CAD build for the part. Positions are in the model's coordinates, mm. Face numbers are marked on the shaded views. A direction names the side the tool comes from. Round coordinates to 2 decimals unless told otherwise and drop trailing zeros. Loops run counter-clockwise (first coordinate to the right, second up) from the corner with the lowest first, then second, coordinate; pieces in that order, holes last. Notation, with made-up numbers: (20.5, -19) - (62.5, -19) arc R33 cw to (62.5, 14) - close; hole circle Ø5 at (83, 54). An arc over 180 degrees is marked (long way). One line per question, with ' | ' between items.
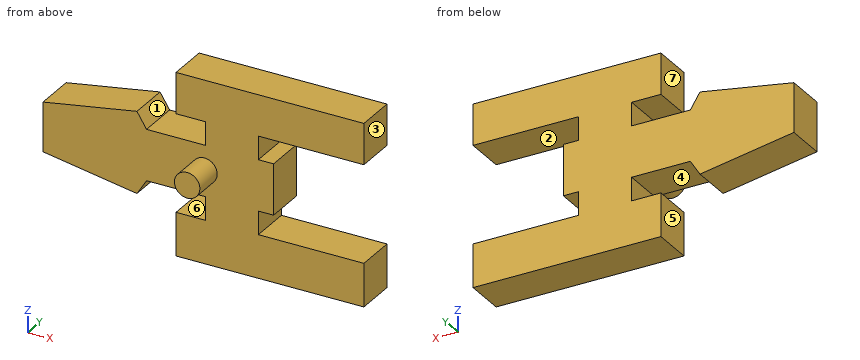
```python
from build123d import *

# Parameters (mm, degrees)
BOSS_EXTRUDE1_DEPTH = 8
SKETCH2_R           = 2.5
BOSS_EXTRUDE2_DEPTH = 6


with BuildPart() as part:
    # Sketch1 → Boss-Extrude1 (new body)
    with BuildSketch(Plane(origin=(0, 0, 0), x_dir=(1, 0, 0), z_dir=(0, 1, 0))):
        Polygon((35.785540038, 49.619336569), (37.676406325, 46.619336569), (49.238802, 46.619336569), (49.238802, 51.219336569), (43.473118302, 51.219336569), (43.473118302, 59.719336569), (80.473118302, 59.719336569), (80.473118302, 51.219336569), (59.689103703, 51.219336569), (59.689103703, 46.619336569), (62.692063962, 46.619336569), (62.692063962, 36.619336569), (59.689103703, 36.619336569), (59.689103703, 32.019336569), (80.473118302, 32.019336569), (80.473118302, 23.971403073), (43.473118302, 23.971403073), (43.473118302, 32.019336569), (49.238802, 32.019336569), (49.238802, 36.619336569), (37.676406325, 36.619336569), (35.785540038, 33.619336569), (17.28730484, 36.774336569), (17.28730484, 46.466988702), align=None)
    extrude(amount=BOSS_EXTRUDE1_DEPTH)

    # Sketch2 → Boss-Extrude2 (add)
    with BuildSketch(Plane.XZ):
        with Locations((49.08730484, -41.619733902)):
            Circle(SKETCH2_R)
    extrude(amount=BOSS_EXTRUDE2_DEPTH)


solid = part.part
```
(1) Cut at B-B, the plane x = 71. Write the cut outline in (y, z).
Results found:
outline: (0, -59.72) - (8, -59.72) - (8, -51.22) - (0, -51.22) - close; (0, -32.02) - (8, -32.02) - (8, -23.97) - (0, -23.97) - close
(2) Two-plate mould, pull along X, no slides. Class the marked faces 1, 2, 3 and 4: released by +X, released by -X, zero draft, split by the parting line, or undercut.
Results found:
face 1: undercut | face 2: zero draft | face 3: released by +X | face 4: undercut
(3) Drop flat-ended pins along their axis: P1, Ø1, axis at x = 44, z = -49.5, coming from the +Y side; P2, Ø4, axis at y = 6, z = -27, coming from the -X side; P3, Ø2, axis at x = 56.5, z = -34, coming from the -Y side; P4, Ø1, axis at y = -1.5, z = -43.5, coming from the -X side. Give the stop position or say it passes through.
Results found:
P1: passes through | P2: stops at x = 43.47 | P3: stops at y = 0 | P4: stops at x = 47
(4) Cut at C-C, the plane z = -48.5. Write the cut outline in (x, y), then the cut area to 3 significant figures.
Results found:
outline: (29.22, 0) - (36.49, 0) - (36.49, 8) - (29.22, 8) - close; (49.24, 0) - (59.69, 0) - (59.69, 8) - (49.24, 8) - close | area: 142 mm²
(5) Tool access for the marked faces 5, 6 and 7: list every direction of +Z, -Z, +X, -X, +Y, -Y with a clear straight run to the whole face (end or side of a thin tool).
Results found:
face 5: -Z, -X, +Y, -Y | face 6: -X, +Y, -Y | face 7: +Z, -X, +Y, -Y
(6) Cut at A-A, the plane x = 45. Write the cut outline in (y, z).
Results found:
outline: (0, -59.72) - (8, -59.72) - (8, -51.22) - (0, -51.22) - close; (0, -46.62) - (8, -46.62) - (8, -36.62) - (0, -36.62) - close; (0, -32.02) - (8, -32.02) - (8, -23.97) - (0, -23.97) - close
(7) Probe L1, parallel to Z at x = 45, y = 0.25; L2, parallel to X at y = 1.5, z = -33.5; L3, parallel to Y at x = 25, z = -36. List the from-to ranges inside material, lowest first.
Results found:
L1: z = -59.72 to -51.22, -46.62 to -36.62, -32.02 to -23.97 | L2: x = 49.24 to 59.69 | L3: y = 0 to 8
(8) Cut at D-D, the plane y = 6.5. Write the cut outline in (x, z).
Results found:
outline: (17.29, -46.47) - (35.79, -49.62) - (37.68, -46.62) - (49.24, -46.62) - (49.24, -51.22) - (43.47, -51.22) - (43.47, -59.72) - (80.47, -59.72) - (80.47, -51.22) - (59.69, -51.22) - (59.69, -46.62) - (62.69, -46.62) - (62.69, -36.62) - (59.69, -36.62) - (59.69, -32.02) - (80.47, -32.02) - (80.47, -23.97) - (43.47, -23.97) - (43.47, -32.02) - (49.24, -32.02) - (49.24, -36.62) - (37.68, -36.62) - (35.79, -33.62) - (17.29, -36.77) - close
